Input: part model. Units: mm. Frame: model coordinates. Face numbers are marked on the shaded views. A direction names the side the tool comes from. Round coordinates to 2 decimals unless told otherwise and drop trailing zeros. Loops run counter-clockwise (first coordinate to the right, second up) from the corner with the lowest first, then second, coordinate; pieces in that order, holes last.
1) Ray query, line 1 along Y through (x, z) = (87.5, 2.3); line 2 along X through (y, z) = (-3, 2.75); line 3 along Y through (x, z) = (92.5, 2.45). Return the intervals inside material, ascending.
2) Section D-D, the plane y = 21.5. Return loops of the section in (x, z).
3) Section B-B, the plane y = 7.5. Return loops of the section in (x, z).
4) Access query for the marked faces 4, 5, 6 and 7. Directions: +Z, -Z, +X, -X, +Y, -Y. A direction counts if a zero-diameter tool reaches every point of the face in a straight line with its end or side. Return the directions, or none.
5) Section C-C, the plane z = 1. State how many separate pieces and enclosed holes the cut face has, and give its area (3 significant figures).
6) Draft query along Y for the marked faces 1, 2 and 3. Return one class per face: pulls with the +Y half, pulls with the -Y half, needs draft (parallel to the pull), parting line crosses it, or undercut.
7) Section A-A, the plane x = 93.25. Return loops of the section in (y, z), and give its area (3 significant figures).
8) First-contact query: pin 1 (0.9 mm diameter, centred on y = 23, z = 2, fed in from +X); pin 2 (1.5 mm diameter, centred on x = 89, z = 1, fed in from +Y); pin 3 (2.5 mm diameter, centred on x = 88.03, y = 4.59, fed in from +Z); pin 4 (1.5 mm diameter, centred on x = 83, z = 2, fed in from -Y). Flat tips, straight axial feed; report the tip coordinate or a pass-through.
from build123d import *

# Parameters (mm, degrees)
ESQUISSE18_R        = 1.5
BOSS_EXTRU_18_DEPTH = 3
CONG_1_R            = 0.3


with BuildPart() as part:
    # Esquisse18 → Boss.-Extru.18 (new body)
    with BuildSketch(Plane.XY):
        with BuildLine():
            Line((97.025632531, 29.590316063), (83.99617235, 16.560855882))
            Line((83.99617235, 16.560855882), (83.99617235, 0.958265781))
            ThreePointArc((83.99617235, 0.958265781), (83.812104956, 0.91607214), (83.639294573, 0.992214643))
            ThreePointArc((83.639294573, 0.992214643), (82.474359337, 1.824587373), (81.150565301, 2.370011808))
            ThreePointArc((81.150565301, 2.370011808), (80.997528298, 2.372778276), (80.863045123, 2.29968756))
            ThreePointArc((80.863045123, 2.29968756), (80.641045132, 2.084165463), (80.425523035, 1.862165472))
            ThreePointArc((80.425523035, 1.862165472), (80.352432318, 1.727682296), (80.355198786, 1.574645294))
            ThreePointArc((80.355198786, 1.574645294), (80.900623221, 0.250851257), (81.732995951, -0.914083979))
            ThreePointArc((81.732995951, -0.914083979), (81.809478339, -1.090727988), (81.76286699, -1.277489987))
            ThreePointArc((81.76286699, -1.277489987), (81.668844739, -1.427698297), (81.578421737, -1.580100401))
            ThreePointArc((81.578421737, -1.580100401), (81.491649145, -1.734610069), (81.408576058, -1.891139882))
            ThreePointArc((81.408576058, -1.891139882), (81.270141097, -2.024887494), (81.078921703, -2.046973808))
            ThreePointArc((81.078921703, -2.046973808), (79.65387183, -1.908585496), (78.234720348, -2.098131098))
            ThreePointArc((78.234720348, -2.098131098), (78.100803182, -2.172253768), (78.020882694, -2.302793773))
            ThreePointArc((78.020882694, -2.302793773), (77.93638611, -2.600441379), (77.860738495, -2.90046006))
            ThreePointArc((77.860738495, -2.90046006), (77.864681666, -3.053471264), (77.943595998, -3.184621962))
            ThreePointArc((77.943595998, -3.184621962), (79.077844433, -4.058349009), (80.38116798, -4.651026153))
            ThreePointArc((80.38116798, -4.651026153), (80.535725676, -4.765763159), (80.588740063, -4.950809468))
            ThreePointArc((80.588740063, -4.950809468), (80.58241856, -5.127904807), (80.580310995, -5.305100401))
            ThreePointArc((80.580310995, -5.305100401), (80.58241856, -5.482295995), (80.588740063, -5.659391333))
            ThreePointArc((80.588740063, -5.659391333), (80.535725676, -5.844437642), (80.38116798, -5.959174648))
            ThreePointArc((80.38116798, -5.959174648), (79.077844433, -6.551851792), (77.943595998, -7.425578839))
            ThreePointArc((77.943595998, -7.425578839), (77.864681666, -7.556729537), (77.860738495, -7.709740741))
            ThreePointArc((77.860738495, -7.709740741), (77.93638611, -8.009759422), (78.020882694, -8.307407028))
            ThreePointArc((78.020882694, -8.307407028), (78.100803182, -8.437947034), (78.234720348, -8.512069703))
            ThreePointArc((78.234720348, -8.512069703), (79.65387183, -8.701615305), (81.078921703, -8.563226993))
            ThreePointArc((81.078921703, -8.563226993), (81.270141097, -8.585313307), (81.408576058, -8.719060919))
            ThreePointArc((81.408576058, -8.719060919), (81.491649145, -8.875590732), (81.578421737, -9.030100401))
            ThreePointArc((81.578421737, -9.030100401), (81.668844739, -9.182502504), (81.76286699, -9.332710814))
            ThreePointArc((81.76286699, -9.332710814), (81.809478339, -9.519472813), (81.732995951, -9.696116822))
            ThreePointArc((81.732995951, -9.696116822), (80.900623221, -10.861052059), (80.355198786, -12.184846095))
            ThreePointArc((80.355198786, -12.184846095), (80.352432318, -12.337883097), (80.425523035, -12.472366273))
            ThreePointArc((80.425523035, -12.472366273), (80.641045132, -12.694366264), (80.863045123, -12.909888361))
            ThreePointArc((80.863045123, -12.909888361), (80.997528298, -12.982979077), (81.150565301, -12.98021261))
            ThreePointArc((81.150565301, -12.98021261), (82.474359337, -12.434788174), (83.639294573, -11.602415444))
            ThreePointArc((83.639294573, -11.602415444), (83.815938583, -11.525933057), (84.002700581, -11.572544405))
            ThreePointArc((84.002700581, -11.572544405), (84.152908892, -11.666566657), (84.305310995, -11.756989659))
            ThreePointArc((84.305310995, -11.756989659), (84.459820663, -11.843762251), (84.616350477, -11.926835338))
            ThreePointArc((84.616350477, -11.926835338), (84.750098088, -12.065270299), (84.772184402, -12.256489692))
            ThreePointArc((84.772184402, -12.256489692), (84.633796091, -13.681539565), (84.823341693, -15.100691048))
            ThreePointArc((84.823341693, -15.100691048), (84.897464362, -15.234608214), (85.028004367, -15.314528702))
            ThreePointArc((85.028004367, -15.314528702), (85.325651974, -15.399025285), (85.625670654, -15.474672901))
            ThreePointArc((85.625670654, -15.474672901), (85.778681859, -15.47072973), (85.909832557, -15.391815398))
            ThreePointArc((85.909832557, -15.391815398), (86.783559604, -14.257566963), (87.376236747, -12.954243415))
            ThreePointArc((87.376236747, -12.954243415), (87.490973753, -12.79968572), (87.676020063, -12.746671333))
            ThreePointArc((87.676020063, -12.746671333), (87.853115401, -12.752992835), (88.030310995, -12.755100401))
            ThreePointArc((88.030310995, -12.755100401), (88.207506589, -12.752992835), (88.384601928, -12.746671333))
            ThreePointArc((88.384601928, -12.746671333), (88.569648237, -12.79968572), (88.684385243, -12.954243415))
            ThreePointArc((88.684385243, -12.954243415), (89.277062386, -14.257566963), (90.150789434, -15.391815398))
            ThreePointArc((90.150789434, -15.391815398), (90.281940131, -15.47072973), (90.434951336, -15.474672901))
            ThreePointArc((90.434951336, -15.474672901), (90.734970016, -15.399025285), (91.032617623, -15.314528702))
            ThreePointArc((91.032617623, -15.314528702), (91.163157628, -15.234608214), (91.237280298, -15.100691048))
            ThreePointArc((91.237280298, -15.100691048), (91.426825899, -13.681539565), (91.288437588, -12.256489692))
            ThreePointArc((91.288437588, -12.256489692), (91.310523902, -12.065270299), (91.444271513, -11.926835338))
            ThreePointArc((91.444271513, -11.926835338), (91.600801327, -11.843762251), (91.755310995, -11.756989659))
            ThreePointArc((91.755310995, -11.756989659), (91.907713098, -11.666566657), (92.057921409, -11.572544405))
            ThreePointArc((92.057921409, -11.572544405), (92.244683407, -11.525933057), (92.421327417, -11.602415444))
            ThreePointArc((92.421327417, -11.602415444), (93.586262653, -12.434788174), (94.91005669, -12.98021261))
            ThreePointArc((94.91005669, -12.98021261), (95.063093692, -12.982979077), (95.197576867, -12.909888361))
            ThreePointArc((95.197576867, -12.909888361), (95.419576859, -12.694366264), (95.635098955, -12.472366273))
            ThreePointArc((95.635098955, -12.472366273), (95.708189672, -12.337883097), (95.705423204, -12.184846095))
            ThreePointArc((95.705423204, -12.184846095), (95.159998769, -10.861052059), (94.327626039, -9.696116822))
            ThreePointArc((94.327626039, -9.696116822), (94.251143651, -9.519472813), (94.297755, -9.332710814))
            ThreePointArc((94.297755, -9.332710814), (94.391777251, -9.182502504), (94.482200253, -9.030100401))
            ThreePointArc((94.482200253, -9.030100401), (94.568972845, -8.875590732), (94.652045932, -8.719060919))
            ThreePointArc((94.652045932, -8.719060919), (94.790480893, -8.585313307), (94.981700287, -8.563226993))
            ThreePointArc((94.981700287, -8.563226993), (96.40675016, -8.701615305), (97.825901643, -8.512069703))
            ThreePointArc((97.825901643, -8.512069703), (97.959818808, -8.437947034), (98.039739296, -8.307407028))
            ThreePointArc((98.039739296, -8.307407028), (98.12423588, -8.009759422), (98.199883495, -7.709740741))
            ThreePointArc((98.199883495, -7.709740741), (98.195940325, -7.556729537), (98.117025992, -7.425578839))
            ThreePointArc((98.117025992, -7.425578839), (96.982777557, -6.551851792), (95.67945401, -5.959174648))
            ThreePointArc((95.67945401, -5.959174648), (95.524896314, -5.844437642), (95.471881927, -5.659391333))
            ThreePointArc((95.471881927, -5.659391333), (95.47820343, -5.482295994), (95.480310995, -5.305100401))
            ThreePointArc((95.480310995, -5.305100401), (95.47820343, -5.127904807), (95.471881927, -4.950809468))
            ThreePointArc((95.471881927, -4.950809468), (95.524896314, -4.765763159), (95.67945401, -4.651026153))
            ThreePointArc((95.67945401, -4.651026153), (96.982777557, -4.058349009), (98.117025992, -3.184621962))
            ThreePointArc((98.117025992, -3.184621962), (98.195940325, -3.053471264), (98.199883495, -2.90046006))
            ThreePointArc((98.199883495, -2.90046006), (98.12423588, -2.600441379), (98.039739296, -2.302793773))
            ThreePointArc((98.039739296, -2.302793773), (97.959818808, -2.172253768), (97.825901643, -2.098131098))
            ThreePointArc((97.825901643, -2.098131098), (96.40675016, -1.908585496), (94.981700287, -2.046973808))
            ThreePointArc((94.981700287, -2.046973808), (94.790480893, -2.024887494), (94.652045932, -1.891139882))
            ThreePointArc((94.652045932, -1.891139882), (94.568972845, -1.734610069), (94.482200253, -1.580100401))
            ThreePointArc((94.482200253, -1.580100401), (94.391777251, -1.427698297), (94.297755, -1.277489987))
            ThreePointArc((94.297755, -1.277489987), (94.251143651, -1.090727988), (94.327626039, -0.914083979))
            ThreePointArc((94.327626039, -0.914083979), (95.159998769, 0.250851257), (95.705423204, 1.574645294))
            ThreePointArc((95.705423204, 1.574645294), (95.708189672, 1.727682296), (95.635098955, 1.862165472))
            ThreePointArc((95.635098955, 1.862165472), (95.419576859, 2.084165463), (95.197576867, 2.29968756))
            ThreePointArc((95.197576867, 2.29968756), (95.063093692, 2.372778276), (94.91005669, 2.370011808))
            ThreePointArc((94.91005669, 2.370011808), (93.586262653, 1.824587373), (92.421327417, 0.992214643))
            ThreePointArc((92.421327417, 0.992214643), (92.244683407, 0.915732256), (92.057921409, 0.962343604))
            ThreePointArc((92.057921409, 0.962343604), (92.032989683, 0.978295443), (92.007994778, 0.994148104))
            Line((92.007994778, 0.994148104), (92.007994778, 14.347176993))
            Line((92.007994778, 14.347176993), (97.025632531, 19.364814746))
            Line((97.025632531, 19.364814746), (97.025632531, 29.590316063))
        make_face()
        with Locations((88.030310995, -5.305100401)):
            Circle(ESQUISSE18_R, mode=Mode.SUBTRACT)
        with Locations((88.030310995, 4.590763304)):
            Circle(ESQUISSE18_R, mode=Mode.SUBTRACT)
    extrude(amount=BOSS_EXTRU_18_DEPTH)

    # Congé1
    cong_1_edges = [part.edges().sort_by_distance(p)[0] for p in [
        (83.99617235, 16.560855882, 1.5),
        (97.025632531, 29.590316063, 1.5),
        (97.025632531, 19.364814746, 1.5),
    ]]
    fillet(cong_1_edges, radius=CONG_1_R)


solid = part.part
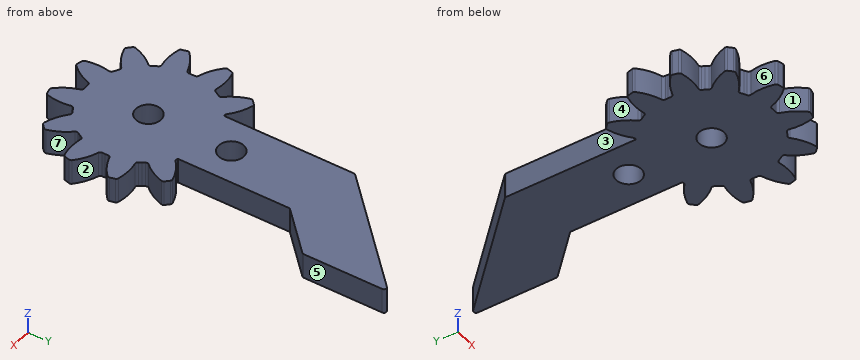
Final values:
1. line 1: y = -12.79 to -6.71, -3.9 to 3.19, 5.99 to 20.06
1. line 2: x = 77.85 to 98.21
1. line 3: y = -11.67 to 1.06, 14.84 to 25.06
2. outline: (88.94, 0) - (97.03, 0) - (97.03, 3) - (88.94, 3) - close
3. outline: (84, 0) - (92.01, 0) - (92.01, 3) - (84, 3) - close
4. face 4: +Z, -Z, -X
4. face 5: +Z, -Z, +X, +Y
4. face 6: +Z, -Z
4. face 7: +Z, -Z, +X
5. separate pieces: 1
5. enclosed holes: 2
5. area: 426 mm2
6. face 1: pulls with the -Y half
6. face 2: undercut
6. face 3: needs draft
7. outline: (-12.23, 0) - (1.62, 0) - (1.62, 3) - (-12.23, 3) - close; (15.59, 0) - (25.81, 0) - (25.81, 3) - (15.59, 3) - close
7. area: 72.3 mm2
8. pin 1: stops at x = 97.03
8. pin 2: stops at y = 22.31
8. pin 3: passes through
8. pin 4: stops at y = -12.55
